Check sheet for the modelled part. Datum: model origin and axes. Units: mm. Face numbers are marked on the shaded views. A direction names the side the tool comes from. Give positions to 0.01 mm unless a question says otherwise; leave off trailing zeros. Order: outer loops, then holes, each group sorted by start corner. A loop starts at its lowest first (then second) coordinate and runs counter-clockwise, first axis right, second up. Notation, with made-up numbers: M -29.5,-4 L -15.5,-4 A8 ccw -15.5,0 Z; hole C -37.5,-30.75 d1. An arc over 180 degrees is marked long. Return JSON: item names as keys, results as strings. Group by question number.
from build123d import *

# Parameters (mm, degrees)
SKETCH_2_R          = 1.7
CUT_EXTRUDE_1_DEPTH = 6
SKETCH_3_R          = 3.25
CUT_EXTRUDE_2_DEPTH = 3.3
SKETCH_4_R          = 4
CUT_EXTRUDE_3_DEPTH = 46


with BuildPart() as part:
    # 草图1 → 旋转1 (revolve)
    with BuildSketch(Plane(origin=(0, 0, 0), x_dir=(1, 0, 0), z_dir=(0, 1, 0))):
        Polygon((0, 0), (0, 16), (-5, 16), (-5, 0), (-45, 0), (-45, -7.5), (0, -7.5), align=None)
    revolve(axis=Axis((0, 0, 7.5), (-1, 0, 0)))

    # 草图2 → 切除-拉伸1 (cut, through all)
    with BuildSketch(Plane.ZY.offset(5)):
        with Locations((7.5, 12)):
            Circle(SKETCH_2_R)
        with Locations((19.5, 0)):
            Circle(SKETCH_2_R)
        with Locations((7.5, -12)):
            Circle(SKETCH_2_R)
        with Locations((-4.5, 0)):
            Circle(SKETCH_2_R)
    extrude(amount=-CUT_EXTRUDE_1_DEPTH, mode=Mode.SUBTRACT)

    # 草图3 → 切除-拉伸2 (cut)
    with BuildSketch(Plane(origin=(0, 0, 0), x_dir=(0, 0, -1), z_dir=(1, 0, 0))):
        with Locations((-7.5, 12)):
            Circle(SKETCH_3_R)
        with Locations((-19.5, 0)):
            Circle(SKETCH_3_R)
        with Locations((4.5, 0)):
            Circle(SKETCH_3_R)
        with Locations((-7.5, -12)):
            Circle(SKETCH_3_R)
    extrude(amount=-CUT_EXTRUDE_2_DEPTH, mode=Mode.SUBTRACT)

    # 草图4 → 切除-拉伸3 (cut, through all)
    with BuildSketch(Plane.ZY.offset(45)):
        with Locations((7.5, 0)):
            Circle(SKETCH_4_R)
    extrude(amount=-CUT_EXTRUDE_3_DEPTH, mode=Mode.SUBTRACT)


solid = part.part
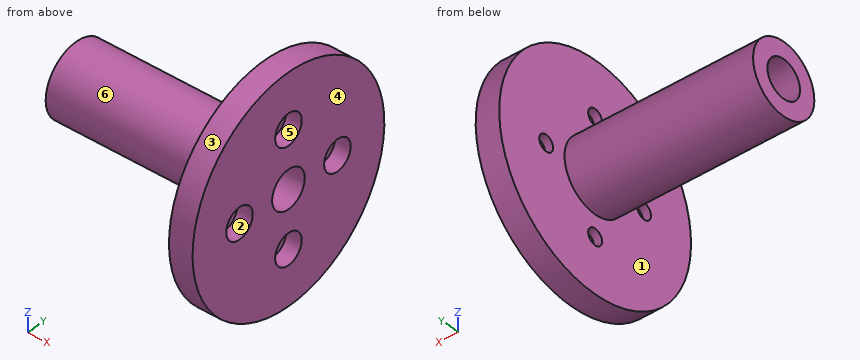
1) Sectioned sample at D-D on y = -2.5. Record the boundary of the cut face in (x, z).
2) Tool access check on the marked faces 1, 2 and 3. Record the directions out of +Z, -Z, +X, -X, +Y, -Y that give a thin tool (end or side, any length) a straight path to the whole face; none if there is none.
3) Sectioned sample at C-C on x = -12. Record the boundary of the cut face in (y, z).
4) Sectioned sample at B-B on y = 12. Record the boundary of the cut face in (x, z), then the cut area to 3 significant figures.
5) Release check for a two-part mould opening along Z. For the marked faces 4, 5 and 6 record: released by +Z, released by -Z, zero draft, split by the parting line, or undercut.
6) Sectioned sample at A-A on z = 7.5. Record the boundary of the cut face in (x, y).
7) Depth check by flat-ended pin: P1, Ø4, axis at y = 12, z = 7.5, coming from the -X side; P2, Ø2, axis at y = -12.5, z = 6.5, coming from the +X side; P3, Ø5, axis at x = -38.5, z = 9.5, coming from the +Y side. Enter the tip coordinate at first touch or a pass-through.
8) Material ranges on line 1 along Y through (x, z) = (-2.3, 7.5); line 2 along Y through (x, z) = (-4.4, 7.5); line 3 along Y through (x, z) = (-20, 7.5), recorded low to high.
Reply:
{
 "1": {"outline": "M -45,0.43 L -5,0.43 L -5,-15.87 L 0,-15.87 L 0,-6.58 L -3.3,-6.58 L -3.3,-2.42 L 0,-2.42 L 0,4.38 L -45,4.38 Z; M -45,10.62 L 0,10.62 L 0,17.42 L -3.3,17.42 L -3.3,21.58 L 0,21.58 L 0,30.87 L -5,30.87 L -5,14.57 L -45,14.57 Z"},
 "2": {"face 1": "-X", "face 2": "+X", "face 3": "+X, -X"},
 "3": {"outline": "C 0,7.5 d15; hole C 0,7.5 d8"},
 "4": {"outline": "M -5,-12.71 L 0,-12.71 L 0,4.25 L -3.3,4.25 L -3.3,5.8 L -5,5.8 Z; M -5,9.2 L -3.3,9.2 L -3.3,10.75 L 0,10.75 L 0,27.71 L -5,27.71 Z", "area": "175 mm^2"},
 "5": {"face 4": "zero draft", "face 5": "undercut", "face 6": "split by the parting line"},
 "6": {"outline": "M -45,-7.5 L -5,-7.5 L -5,-10.3 L -3.3,-10.3 L -3.3,-8.75 L 0,-8.75 L 0,-4 L -45,-4 Z; M -45,4 L 0,4 L 0,8.75 L -3.3,8.75 L -3.3,10.3 L -5,10.3 L -5,7.5 L -45,7.5 Z; M -5,-23.5 L 0,-23.5 L 0,-15.25 L -3.3,-15.25 L -3.3,-13.7 L -5,-13.7 Z; M -5,13.7 L -3.3,13.7 L -3.3,15.25 L 0,15.25 L 0,23.5 L -5,23.5 Z"},
 "7": {"P1": "x = -5", "P2": "x = -3.3", "P3": "y = 7.5"},
 "8": {"line 1": "-23.5 to -15.25, -8.75 to -4, 4 to 8.75, 15.25 to 23.5", "line 2": "-23.5 to -13.7, -10.3 to -4, 4 to 10.3, 13.7 to 23.5", "line 3": "-7.5 to -4, 4 to 7.5"}
}
